Print and shaded views of the part. All mm, measured from the part's lowest x, y and z. A direction names the side the tool comes from. Give positions to 0.01 mm unless a question says otherwise; leave off trailing zeros. Order: outer loops, then holes, each group sorted by start corner. A loop starts at its lowest first (then second) coordinate and runs counter-clockwise, first axis right, second up. Notation, with made-up numbers: (-38, 17.5) - (-5, 17.5) arc R19 cw to (-5, 38.5) - close; hole circle Ø1 at (51, -7.5). An arc over 180 degrees is marked (long way). Answer in a Markdown table with one row per item.
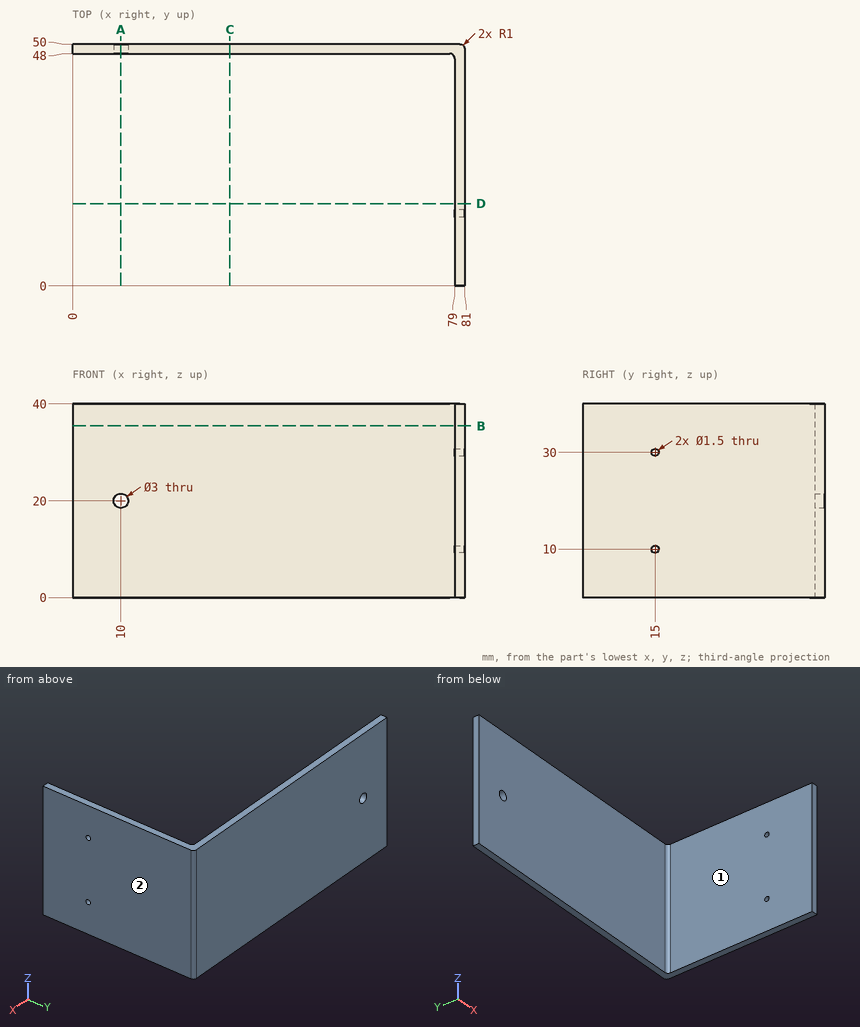
1. Probe line 1 (Z direction, x = 79.4, y = 15); line 2 (Y direction, x = 80, z = 10); line 3 (X direction, y = 48.4, z = 20). List the from-to ranges inside material, lowest first.
Check result:
| item | result |
|---|---|
| line 1 | z = 0 to 9.25, 10.75 to 29.25, 30.75 to 40 |
| line 2 | y = 0 to 14.25, 15.75 to 50 |
| line 3 | x = 0 to 8.5, 11.5 to 81 |
2. Cut at D-D on y = 17. Write the cut outline in (x, z), and give its area (3 significant figures).
Check result:
| item | result |
|---|---|
| outline | (79, 0) - (81, 0) - (81, 40) - (79, 40) - close |
| area | 80.0 mm² |
3. Cut at A-A on x = 10. Write the cut outline in (y, z).
Check result:
| item | result |
|---|---|
| outline | (48, 0) - (50, 0) - (50, 18.5) - (48, 18.5) - close; (48, 21.5) - (50, 21.5) - (50, 40) - (48, 40) - close |
4. Drop flat-ended pins along their axis: P1, Ø2.5, axis at x = 10, z = 20, coming from the -Y side; P2, Ø12, axis at y = 19.5, z = 28.5, coming from the -X side. Give the stop position or say it passes through.
Check result:
| item | result |
|---|---|
| P1 | passes through |
| P2 | stops at x = 79 |
5. Which spindle directions (+Z, -Z, +X, -X, +Y, -Y) get a long thin tool onto all of the face, cutting with end or side? Do the marked faces 1 and 2. Say none if no direction does.
Check result:
| item | result |
|---|---|
| face 1 | +Z, -Z, -X, -Y |
| face 2 | +Z, -Z, +X, +Y, -Y |
6. Cut at B-B on z = 35.5. Write the cut outline in (x, y).
Check result:
| item | result |
|---|---|
| outline | (0, 48) - (78, 48) arc R1 cw to (79, 47) - (79, 0) - (81, 0) - (81, 49) arc R1 ccw to (80, 50) - (0, 50) - close |
7. Cut at C-C on x = 32.5. Write the cut outline in (y, z).
Check result:
| item | result |
|---|---|
| outline | (48, 0) - (50, 0) - (50, 40) - (48, 40) - close |
